from build123d import *

# Parameters (mm, degrees)
SKETCH1_W                = 43.18
SKETCH1_H                = 17.78
SKETCH1_R                = 0.83
BOSS_EXTRUDE1_DEPTH      = 1.57
SKETCH2_W                = 10
SKETCH2_H                = 10
BOSS_EXTRUDE2_DEPTH      = 2
CHAMFER1_SIZE            = 0.5
BOSS_EXTRUDE3_DEPTH      = 1
BOSS_EXTRUDE3_DEPTH_BACK = 5
SKETCH4_W                = 2.380224585
SKETCH4_H                = 2.317587096
SKETCH4_W_2              = 1.628574716
SKETCH4_H_2              = 3.570336877
SKETCH4_W_3              = 4.823086659
SKETCH4_H_3              = 5.950561462
SKETCH4_W_4              = 1.440662249
SKETCH4_H_4              = 0.375824935
BOSS_EXTRUDE4_DEPTH      = 1


with BuildPart() as part:
    # Sketch1 → Boss-Extrude1 (new body)
    with BuildSketch(Plane(origin=(0, 0, 0), x_dir=(1, 0, 0), z_dir=(0, 1, 0))):
        Rectangle(SKETCH1_W, SKETCH1_H)
        with Locations((-20.32, 7.62)):
            Circle(SKETCH1_R, mode=Mode.SUBTRACT)
        with Locations((20.32, 7.62)):
            Circle(SKETCH1_R, mode=Mode.SUBTRACT)
        with Locations((20.32, -7.62)):
            Circle(SKETCH1_R, mode=Mode.SUBTRACT)
        with Locations((-20.32, -7.62)):
            Circle(SKETCH1_R, mode=Mode.SUBTRACT)
    extrude(amount=BOSS_EXTRUDE1_DEPTH)

    # Sketch2 → Boss-Extrude2 (add)
    with BuildSketch(Plane(origin=(0, 1.57, 0), x_dir=(1, 0, 0), z_dir=(0, 1, 0))):
        with Locations((14.59, 0)):
            Rectangle(SKETCH2_W, SKETCH2_H)
    extrude(amount=BOSS_EXTRUDE2_DEPTH)

    # Chamfer1
    chamfer1_edges = [part.edges().sort_by_distance(p)[0] for p in [
        (9.59, 3.57, 0),
        (14.59, 3.57, 5),
        (19.59, 3.57, 0),
        (14.59, 3.57, -5),
    ]]
    chamfer(chamfer1_edges, length=CHAMFER1_SIZE)

    # Sketch3 → Boss-Extrude3 (add, two sides)
    with BuildSketch(Plane.ZY.offset(21.59)) as boss_extrude3_sk:
        with BuildLine():
            Line((-2, 4.07), (2, 4.07))
            ThreePointArc((2, 4.07), (3.25, 2.82), (2, 1.57))
            Line((2, 1.57), (-2, 1.57))
            ThreePointArc((-2, 1.57), (-3.25, 2.82), (-2, 4.07))
        make_face()
    extrude(amount=BOSS_EXTRUDE3_DEPTH)
    extrude(boss_extrude3_sk.sketch, amount=-BOSS_EXTRUDE3_DEPTH_BACK)

    # Sketch4 → Boss-Extrude4 (add)
    with BuildSketch(Plane(origin=(0, 1.57, 0), x_dir=(1, 0, 0), z_dir=(0, 1, 0))):
        with Locations((-14.788997849, 4.667413541)):
            Rectangle(SKETCH4_W, SKETCH4_H)
        with Locations((-14.480791416, -3.105550682)):
            Rectangle(SKETCH4_W_2, SKETCH4_H_2)
        with Locations((-7.750249949, 1.110525399)):
            Rectangle(SKETCH4_W_3, SKETCH4_H_3)
        with Locations((-12.189542052, 1.441582853)):
            Rectangle(SKETCH4_W_4, SKETCH4_H_4)
    extrude(amount=BOSS_EXTRUDE4_DEPTH)


solid = part.part
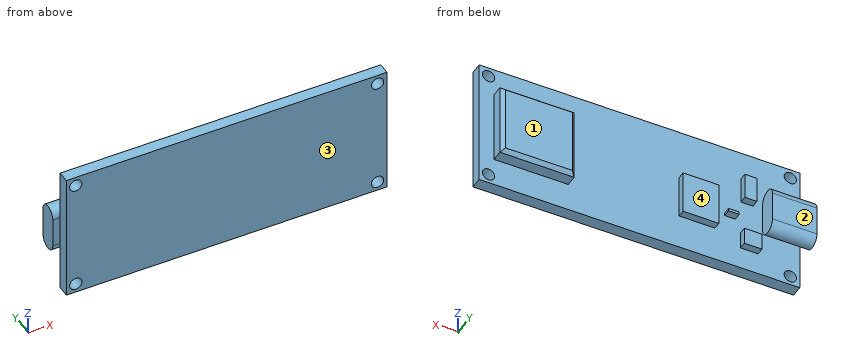
The model under review builds one solid part; all positions refer to its coordinate system, in mm. Face numbers are marked on the shaded views. A direction names the side the tool comes from. Give positions to 0.01 mm unless a question says otherwise; leave off trailing zeros. Order: outer loops, then holes, each group sorted by start corner. A loop starts at its lowest first (then second) coordinate and runs counter-clockwise, first axis right, second up. Notation, with made-up numbers: M 58,69.5 L 102,69.5 A25 ccw 102,100.5 Z; hole C 27.5,19 d9. An arc over 180 degrees is marked long. One line per question, with ' | ' between items. Start each with the question number.
1) Consider section C-C, the plane x = -20.32. Give the boundary of the cut face in (y, z), then the cut area to 3 significant figures.
2) Mouldability with a two-part tool opening along X and no side actions: class the marked faces 3 and 4 as pulls with the +X half, pulls with the -X half, needs draft (parallel to the pull), parting line crosses it, or undercut.
3) Clearance check with flat-ended pins moving along their axes: P1, Ø1, axis at x = 2, z = 4, coming from the -Y side; P2, Ø1, axis at x = -10.5, z = 3, coming from the +Y side; P3, Ø1.1, axis at y = 2, z = 4, coming from the -X side; P4, Ø8, axis at x = 16.5, z = 6.5, coming from the +Y side. State where each tip first meets the part, or that it passes through.
4) Consider section A-A, the plane y = 0.6. Give the boundary of the cut face in (x, z).
5) Consider section B-B, the plane z = 7.62. Give the boundary of the cut face in (x, y), then the cut area to 3 significant figures.
6) For the marked faces 1 and 2, list the 3-axis set-ups (+Z, -Z, +X, -X, +Y, -Y) from which the entire face can be reached by the end or side of a thin tool; tool diameter is ignored.
7) Wall thickness on L1, parallel to Z at x = -20.32, y = 1.15; L2, parallel to X at y = 0.75, z = -7.62; L3, parallel to X at y = 2.1, z = -2.5: over which ranges is each line inside the solid? List them lowest first. Write a range as from..to.
8) Consider section D-D, the plane x = 11. Give the boundary of the cut face in (y, z), then the cut area to 3 significant figures.
Found:
1) outline: M 0,-8.89 L 1.57,-8.89 L 1.57,-8.45 L 0,-8.45 Z; M 0,-6.79 L 1.57,-6.79 L 1.57,-2 A1.25 ccw 4.07,-2 L 4.07,2 A1.25 ccw 1.57,2 L 1.57,6.79 L 0,6.79 Z; M 0,8.45 L 1.57,8.45 L 1.57,8.89 L 0,8.89 Z | area: 37.6 mm²
2) face 3: needs draft | face 4: undercut
3) P1: stops at y = 0 | P2: stops at y = 1.57 | P3: stops at x = -21.59 | P4: stops at y = 3.57
4) outline: M -21.59,-8.89 L 21.59,-8.89 L 21.59,8.89 L -21.59,8.89 Z; hole C -20.32,-7.62 d1.66; hole C -20.32,7.62 d1.66; hole C 20.32,-7.62 d1.66; hole C 20.32,7.62 d1.66
5) outline: M -21.59,0 L -21.15,0 L -21.15,1.57 L -21.59,1.57 Z; M -19.49,0 L 19.49,0 L 19.49,1.57 L -19.49,1.57 Z; M 21.15,0 L 21.59,0 L 21.59,1.57 L 21.15,1.57 Z | area: 62.6 mm²
6) face 1: +Z, -Z, +X, +Y | face 2: +Z, -Z, +X, -X, +Y
7) L1: z = -8.89..-8.45, -6.79..6.79, 8.45..8.89 | L2: x = -21.59..-21.15, -19.49..19.49, 21.15..21.59 | L3: x = -22.59..-16.59, -10.16..-5.34, 9.59..19.59
8) outline: M 0,-8.89 L 1.57,-8.89 L 1.57,-5 L 3.07,-5 L 3.57,-4.5 L 3.57,4.5 L 3.07,5 L 1.57,5 L 1.57,8.89 L 0,8.89 Z | area: 47.7 mm²
